Solid Edge part; units mm, degrees
sketch "Sketch1" plane through (0, 0, 0) normal (0, 0, 1) x (1, 0, 0)
  circle A0 centre (52.9233, 75.7004) radius 85
extrude "Protrusion1" add sketch "Sketch1" along normal blind 4
hole "Furo_1" at (52.9233, 75.7004, 4) direction (0, 0, -1) diameter 10 end up to next
hole "Furo_2" at (52.9233, 75.7004, 4) direction (0, 0, -1) diameter 23 end up to next
hole "Furo_3" at (38.4233, 80.9504, 4) direction (0, 0, -1) diameter 3 end up to next
hole "Hole1" at (38.4233, 70.4504, 4) direction (0, 0, -1) diameter 3 end up to next
hole "Furo_5" at (86.4233, 80.9504, 4) direction (0, 0, -1) diameter 3 end up to next
hole "Hole2" at (86.4233, 70.4504, 4) direction (0, 0, -1) diameter 3 end up to next
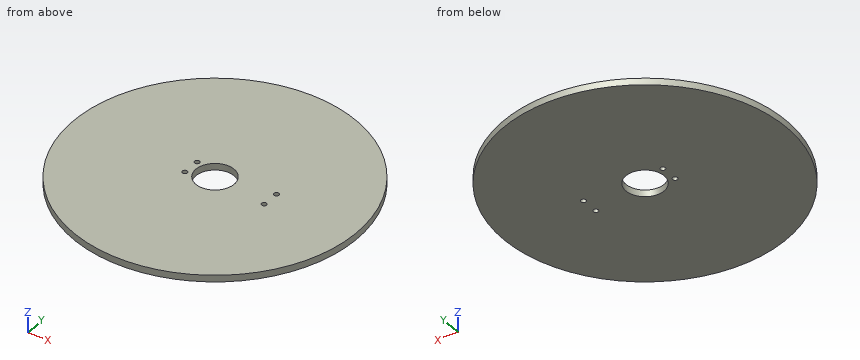
Input: part model. Units: mm. Frame: model coordinates. Give positions to 0.01 mm unless a question says otherwise; leave off trailing zeros. Order: outer loops, then holes, each group sorted by start corner. A loop starts at its lowest first (then second) coordinate and runs counter-clockwise, first axis right, second up. Notation, with made-up numbers: (-34.5, 35) -> (-21.5, 35) arc R26 cw to (-21.5, 54) -> close; hole circle Ø9 at (32, 35). An arc over 180 degrees is marked (long way). Write each question's results on one line, items separated by ' | '. Start each with the question number.
Item 1: Contact query for flat-ended pins moving along their axis: P1, Ø2, axis at y = 109.5, z = 1, coming from the +X side; P2, Ø2, axis at x = 113.5, z = 2.5, coming from the -Y side. Output: stop coordinate, or through.
Item 2: Cut plane D-D on x = 99.5. Return the cut outline in (y, z), then the cut area to 3 significant figures.
Item 3: Cut plane A-A on x = 48.5. Return the cut outline in (y, z), then the cut area to 3 significant figures.
Item 4: Line query: line 1 (X direction, y = 76.5, z = 0.3); line 2 (X direction, y = 69.5, z = 2.9); line 3 (Y direction, x = 37.5, z = 1.25). Output: solid intervals per line, ascending.
Item 5: Cut plane C-C on y = 123. Return the cut outline in (x, z), then the cut area to 3 significant figures.
Item 6: Cut plane B-B on z = 2.5. Return the cut outline in (x, y), then the cut area to 3 significant figures.
Established:
1) P1: x = 131.34 | P2: y = 15.07
2) outline: (4.6, 0) -> (146.8, 0) -> (146.8, 4) -> (4.6, 4) -> close | area: 569 mm^2
3) outline: (-9.18, 0) -> (65.09, 0) -> (65.09, 4) -> (-9.18, 4) -> close; (86.32, 0) -> (160.59, 0) -> (160.59, 4) -> (86.32, 4) -> close | area: 594 mm^2
4) line 1: -32.07 to 41.45, 64.4 to 137.92 | line 2: -31.85 to 37.26, 39.58 to 43.24, 62.61 to 85.26, 87.58 to 137.7 | line 3: -7.89 to 69.27, 71.63 to 79.77, 82.13 to 159.29
5) outline: (-17.7, 0) -> (123.55, 0) -> (123.55, 4) -> (-17.7, 4) -> close | area: 565 mm^2
6) outline: circle Ø170 at (52.92, 75.7); hole circle Ø3 at (38.42, 70.45); hole circle Ø3 at (38.42, 80.95); hole circle Ø23 at (52.92, 75.7); hole circle Ø3 at (86.42, 70.45); hole circle Ø3 at (86.42, 80.95) | area: 22,300 mm^2
